Check sheet for the modelled part. Datum: model origin and axes. Units: mm. A direction names the side the tool comes from. Round coordinates to 2 decimals unless told otherwise and drop trailing zeros. Write each loop counter-clockwise with the first axis right and the second up, starting at its lowest first coordinate (ties: lowest second). Pieces come first, ordered by that corner, then holes. Notation, with made-up numbers: M 32.25,-33 L 66.25,-33 A22 ccw 66.25,-18 Z; hole C 30.5,-31 d4. An arc over 180 degrees is marked long. Answer in a Markdown table with one row per item.
Autodesk Inventor part; units mm, degrees
ref_plane "YZ Plane" through (0, 0, 0) normal (1, 0, 0) x (0, 1, 0)
ref_plane "XZ Plane" through (0, 0, 0) normal (0, 1, 0) x (-1, 0, 0)
ref_plane "XY Plane" through (0, 0, 0) normal (0, 0, 1) x (1, 0, 0)
sketch "スケッチ1" plane through (0, 0, 0) normal (0, 1, 0) x (-1, 0, 0)
  line L0 (0, 0) -> (-5, 0)
  line L1 (-5, 0) -> (-5, 2.8)
  line L2 (-5, 2.8) -> (-3, 2.8)
  line L3 (-3, 2.8) -> (-3, 13.8)
  line L4 (-3, 13.8) -> (-2, 13.8)
  line L5 (-2, 13.8) -> (-2, 21.37)
  line L6 (-1.57, 21.8) -> (0, 21.8)
  line L7 (0, 21.8) -> (0, 0)
  line L8 (-1.57, 21.8) -> (-2, 21.37)
  point P0 (-2, 21.8)
  dimension "d0" = 8
  dimension "d1" = 11
  dimension "d2" = 2.8
  dimension "d3" = 0.43
  dimension "d4" = 0.43
  dimension "d5" = 4
  dimension "d6" = 10
  dimension "d7" = 6
revolve "回転1" add sketch "スケッチ1" angle 360 about axis through (0, 0, 21.8) along (0, 0, -1)
thread "ねじ1"
sketch "スケッチ2" plane through (0, 0, 0) normal (0, 0, -1) x (-1, 0, 0)
  line L0 (0, -1.4434) -> (-1.25, -0.7217)
  line L1 (-1.25, -0.7217) -> (-1.25, 0.7217)
  line L2 (-1.25, 0.7217) -> (0, 1.4434)
  line L3 (0, 1.4434) -> (1.25, 0.7217)
  line L4 (1.25, 0.7217) -> (1.25, -0.7217)
  line L5 (1.25, -0.7217) -> (0, -1.4434)
  point P0 (0, 0)
  point P1 (0, 0)
  dimension "d11" = 2.5
extrude "押し出し1" cut sketch "スケッチ2" against normal blind 1.5
properties part number "DBTS4-11-8-DHC" material "ステンレス鋼 AISI 304"
1. Access from +Z, -Z, +X, -X, +Y, -Y to the whole of each face (thin tool, end or side, straight path). Record for faces 1 (the face through (1, 2, 13.8)), 2 (the face through (0.63, 1.08, 0.74)), 3 (the face through (1.04, 1.04, 0)).
Found:
| item | result |
|---|---|
| face 1 | +Z |
| face 2 | -Z |
| face 3 | -Z, +X, -X, +Y, -Y |
2. Draft check along Y on faces 4 (the face through (-3, 0, 8)), 5 (the face through (0, 0, 1.5)), 6 (the face through (3.3, -0.1, 2.8)). Enter one of: +Y half, -Y half, draft (parallel to the pull), parting line (faces both ways), or undercut.
Found:
| item | result |
|---|---|
| face 4 | parting line |
| face 5 | undercut |
| face 6 | draft |
3. Scan lines: L1, parallel to Z at x = 3.25, y = 0.5; L2, parallel to Z at x = 1.25, y = 1.75; L3, parallel to X at y = 0, z = 12. Record each from-to range of solid material in increasing order.
Found:
| item | result |
|---|---|
| L1 | z = 0 to 2.8 |
| L2 | z = 0 to 13.8 |
| L3 | x = -3 to 3 |
4. Section check C-C, the plane x = -4.5. Record the cut outline in (y, z), and give its area (3 significant figures).
Found:
| item | result |
|---|---|
| outline | M -2.18,0 L 2.18,0 L 2.18,2.8 L -2.18,2.8 Z |
| area | 12.2 mm2 |
5. Section check D-D, the plane z = 20.25. Record the cut outline in (x, y), and give its area (3 significant figures).
Found:
| item | result |
|---|---|
| outline | C 0,0 d4 |
| area | 12.6 mm2 |
6. Section check A-A, the plane y = 0. Record the cut outline in (x, z), and give its area (3 significant figures).
Found:
| item | result |
|---|---|
| outline | M -5,0 L -1.25,0 L -1.25,1.5 L 1.25,1.5 L 1.25,0 L 5,0 L 5,2.8 L 3,2.8 L 3,13.8 L 2,13.8 L 2,21.37 L 1.57,21.8 L -1.57,21.8 L -2,21.37 L -2,13.8 L -3,13.8 L -3,2.8 L -5,2.8 Z |
| area | 122 mm2 |
7. Section check B-B, the plane z = 6.5. Record the cut outline in (x, y), and give its area (3 significant figures).
Found:
| item | result |
|---|---|
| outline | C 0,0 d6 |
| area | 28.3 mm2 |
8. Go/stop test with flat-tipped pins: pin 1 (6 mm diameter, centred on y = 0, z = 13.5, fed in from -X); pin 2 (3 mm diameter, centred on x = -3.5, z = 5, fed in from -Y); pin 3 (1 mm diameter, centred on x = -2.5, z = 10.5, fed in from +Y). Record where each tip stops, or that it passes through.
Found:
| item | result |
|---|---|
| pin 1 | stops at x = -3 |
| pin 2 | stops at y = -2.24 |
| pin 3 | stops at y = 2.24 |
